The drawing under review shows one solid part. Ordinate dimensions are in mm from its lowest x, y, z. A direction names the side the tool comes from. Give positions to 0.01 mm unless a question says otherwise; leave off trailing zeros. Order: outer loops, then holes, each group sorted by start corner. A loop starts at its lowest first (then second) coordinate and runs counter-clockwise, first axis right, second up. Notation, with made-up numbers: (41.5, -6) -> (77.5, -6) arc R13 cw to (77.5, 1) -> close; hole circle Ø7 at (39, 41.25). An arc over 180 degrees is marked (long way). One line per item, written item: value.
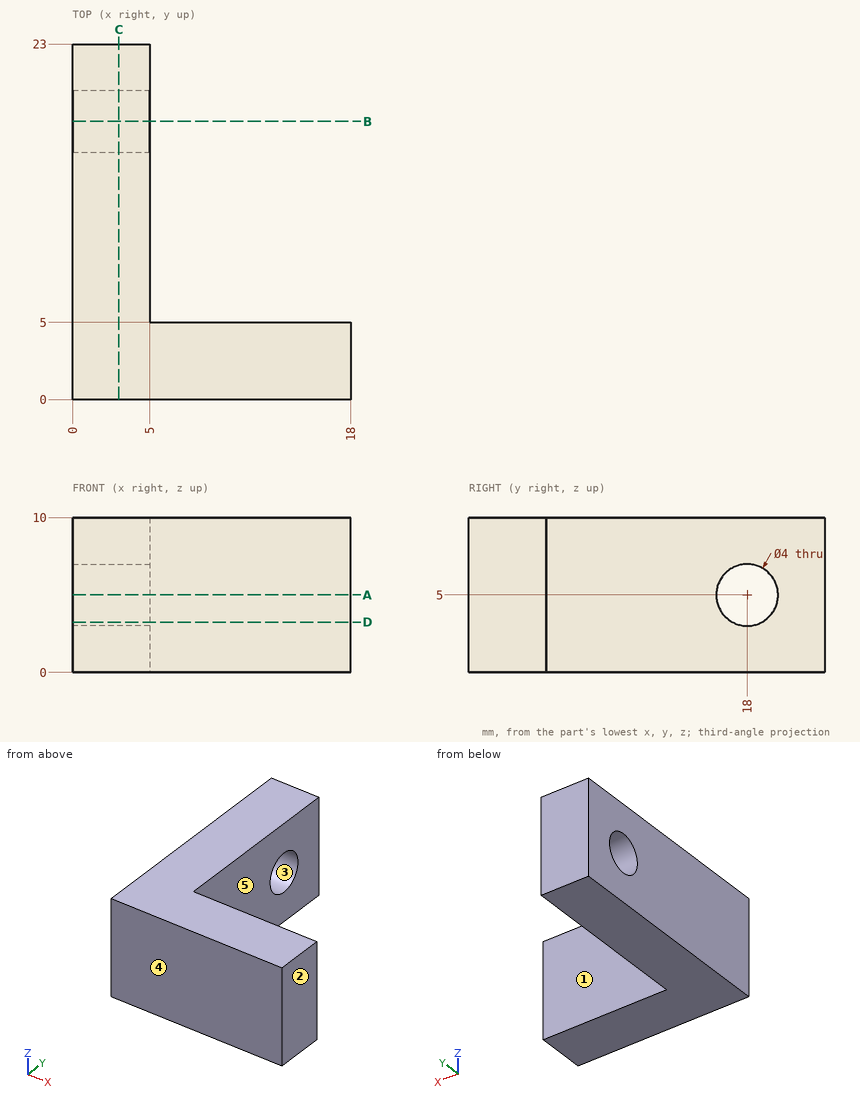
Item 1: To check wall thickness, follow line 1 along Y through (x, z) = (1.6, 5); line 2 along X through (y, z) = (19, 2.25). State the ranges of each line that lie inside material, in increasing order. Write a range as from..to.
Returned:
line 1: 0..16, 20..23
line 2: 0..5
Item 2: Add section C-C on x = 3. Give the boundary of the cut face in (y, z), plus the area to 3 significant figures.
Returned:
outline: (0, 0) -> (23, 0) -> (23, 10) -> (0, 10) -> close; hole circle Ø4 at (18, 5)
area: 217 mm²
Item 3: Add section A-A on z = 5. Give the boundary of the cut face in (x, y), plus the area to 3 significant figures.
Returned:
outline: (0, 0) -> (18, 0) -> (18, 5) -> (5, 5) -> (5, 16) -> (0, 16) -> close; (0, 20) -> (5, 20) -> (5, 23) -> (0, 23) -> close
area: 160 mm²
Item 4: Add section B-B on y = 18. Give the boundary of the cut face in (x, z), plus the area to 3 significant figures.
Returned:
outline: (0, 0) -> (5, 0) -> (5, 3) -> (0, 3) -> close; (0, 7) -> (5, 7) -> (5, 10) -> (0, 10) -> close
area: 30.0 mm²
Item 5: Draft analysis for pull direction Y (two halves, no side actions). For the marked faces 3, 4 and 5, state which applies: pulls with the +Y half, pulls with the -Y half, needs draft (parallel to the pull), parting line crosses it, or undercut.
Returned:
face 3: undercut
face 4: pulls with the -Y half
face 5: needs draft
Item 6: Machinability: for the marked faces 1 and 2, which of the approach directions +Z, -Z, +X, -X, +Y, -Y give a long, thin tool a straight path to every point of the face, cutting with its end or side? Answer none if there is none.
Returned:
face 1: +Z, -Z, +X, +Y
face 2: +Z, -Z, +X, +Y, -Y
Item 7: Clearance check with flat-ended pins moving along their axes: P1, Ø1, axis at x = 3.5, z = 6, coming from the -Y side; P2, Ø5, axis at y = 10.5, z = 3, coming from the +X side; P3, Ø5, axis at x = 12.5, z = 4, coming from the +Y side; P4, Ø3.5, axis at y = 18, z = 5, coming from the -X side. State where each tip first meets the part, or that it passes through.
Returned:
P1: y = 0
P2: x = 5
P3: y = 5
P4: through
Item 8: Add section D-D on z = 3.25. Give the boundary of the cut face in (x, y), plus the area to 3 significant figures.
Returned:
outline: (0, 0) -> (18, 0) -> (18, 5) -> (5, 5) -> (5, 17.03) -> (0, 17.03) -> close; (0, 18.97) -> (5, 18.97) -> (5, 23) -> (0, 23) -> close
area: 170 mm²
